Here's the drawing with two shaded views (mm, measured from the low corner). I have some questions. A direction names the side the tool comes from. Round coordinates to 2 decimals unless told otherwise and drop trailing zeros. Loops run counter-clockwise (first coordinate to the right, second up) from the corner with the lowest first, then second, coordinate; pieces in that order, holes last. Notation, with made-up numbers: (65, 27.5) -> (108, 27.5) arc R15 cw to (108, 44.5) -> close; hole circle Ø11 at (-23.75, -20.5). An arc over 180 degrees is marked (long way). Write each question's results on one line, items separated by ' | '. Start each with the question number.
1) Imagine slicing it at D-D, the plane y = 5.75. List the corners of the cut face in (x, z) for me.
2) If I drill on probe 1 along Y at (x, z) = (7, 4.5); probe 2 along Y at (x, z) = (3.5, 1.5); probe 3 along X at (y, z) = (1, 4.5), over which ranges is the centre line in solid material (lowest first)?
3) Imagine slicing it at A-A, the plane y = 1. List the corners of the cut face in (x, z) for me, plus the area to 3 significant figures.
4) Which directions (+Z, -Z, +X, -X, +Y, -Y) give clear straight access to the entire face, cutting with the end or side of a thin tool? Please do the marked faces 5, 6, 7, 8 and 9.
5) Imagine slicing it at B-B, the plane x = 7.5. List the corners of the cut face in (y, z) for me, plus the area to 3 significant figures.
6) We'd pull the mould along Y, two halves only. Please class the marked faces 1, 2, 3 and 4: pulls with the +Y half, pulls with the -Y half, needs draft (parallel to the pull), parting line crosses it, or undercut.
7) For P1, Ø3, axis at y = 4, z = 7.5, coming from the +X side; P2, Ø0.8, axis at y = 2, z = 6.5, coming from the -X side; P3, Ø4, axis at x = 13.5, y = 6.5, coming from the -Z side (1 decimal), each with a flat end and sliding along its axis, tell me the tip position at first contact or that it passes through.
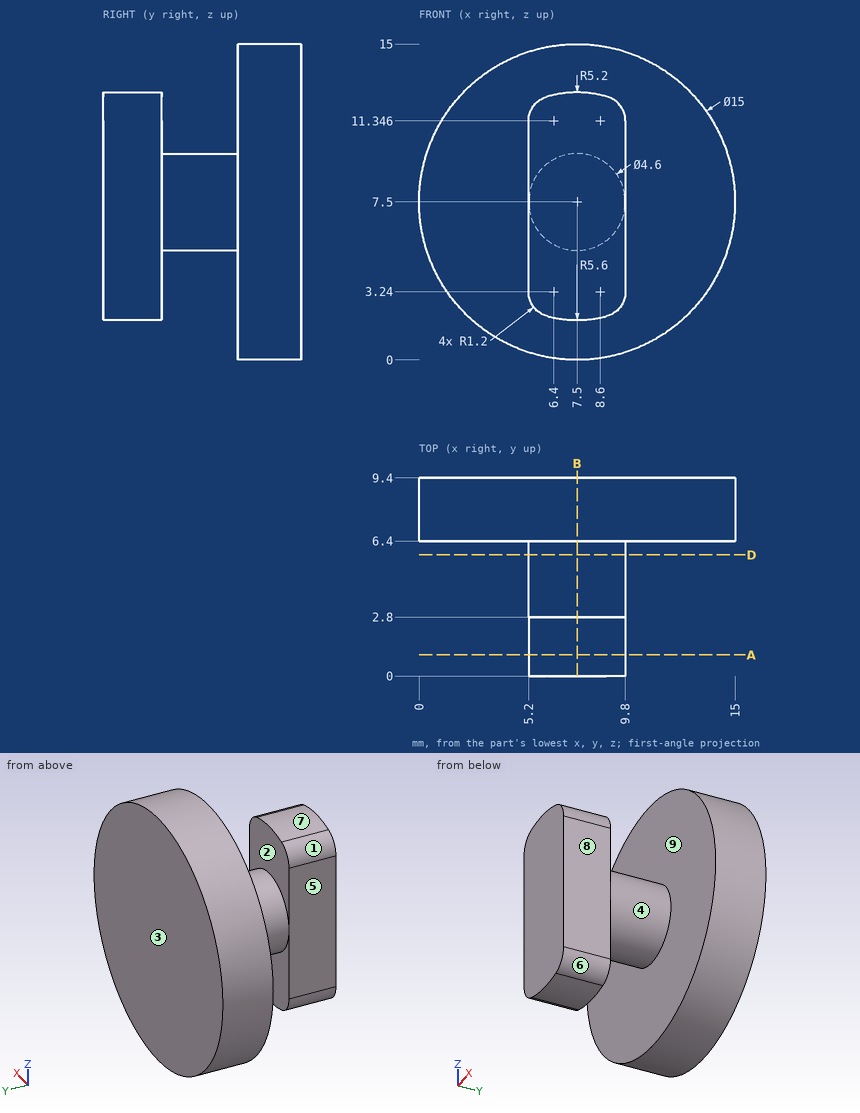
Checked values:
1) outline: circle Ø4.6 at (7.5, 7.5)
2) probe 1: 0 to 2.8, 6.4 to 9.4 | probe 2: 6.4 to 9.4 | probe 3: 5.2 to 9.8
3) outline: (5.2, 3.24) arc R1.2 ccw to (6.1, 2.08) arc R5.6 ccw to (8.9, 2.08) arc R1.2 ccw to (9.8, 3.24) -> (9.8, 11.35) arc R1.2 ccw to (8.93, 12.5) arc R5.2 ccw to (6.07, 12.5) arc R1.2 ccw to (5.2, 11.35) -> close | area: 47.6 mm^2
4) face 5: +Z, -Z, -X, -Y | face 6: -Z, +X, -Y | face 7: +Z, -Y | face 8: +Z, -Z, +X, -Y | face 9: none
5) outline: (0, 1.9) -> (2.8, 1.9) -> (2.8, 5.2) -> (6.4, 5.2) -> (6.4, 0) -> (9.4, 0) -> (9.4, 15) -> (6.4, 15) -> (6.4, 9.8) -> (2.8, 9.8) -> (2.8, 12.7) -> (0, 12.7) -> close | area: 91.8 mm^2
6) face 1: needs draft | face 2: undercut | face 3: pulls with the +Y half | face 4: undercut
7) P1: x = 9.8 | P2: x = 5.2 | P3: z = 1.2
